The listing builds one solid part. Answer for the finished solid, in the listing's coordinates (mm). A direction names the side the tool comes from. Coordinates: 2 decimals unless noted, no trailing zeros. Order: outer loops, then holes, each group sorted by start corner. A loop starts at its lowest first (then second) coordinate and runs counter-clockwise, first axis right, second up.
```python
from build123d import *

# Parameters (mm, degrees)
SKETCH1_W           = 22.5
SKETCH1_H           = 12.2
BOSS_EXTRUDE1_DEPTH = 3.000000026


with BuildPart() as part:
    # Sketch1 → Boss-Extrude1 (new body)
    with BuildSketch(Plane(origin=(3.000000026, 0, 0), x_dir=(0, 0, -1), z_dir=(1, 0, 0))):
        Polygon((-21.320657805, 14.036174864), (-22.758102044, 12.659284286), (-24.039382115, 11.136000976), (-25.149684399, 9.483940899), (-26.076165959, 7.722207811), (-26.808116585, 5.871174857), (-27.337068692, 3.952247556), (-27.656905353, 1.987616299), (-27.763931081, 0), (-27.656905353, -1.987616299), (-27.337068692, -3.952247556), (-26.808116585, -5.871174857), (-26.076165959, -7.722207811), (-25.149684399, -9.483940899), (-24.039382115, -11.136000976), (-22.758102044, -12.659284286), (-21.320657805, -14.036174864), (-19.743673503, -15.250750817), (-18.045384437, -16.28896594), (-16.245434061, -17.138814554), (-14.364630915, -17.790470272), (-12.424727902, -18.236396834), (-7.814312354, -19.272558391), (-3.327161307, -20.754124969), (0.993806054, -22.666925564), (5.107260309, -24.992663413), (8.973857388, -27.709092945), (12.55661156, -30.790233985), (15.821257606, -34.206613898), (22.763932127, -34.206613898), (22.763932127, -28.999887407), (27.763931084, -28.999887407), (27.763931084, -18.99988763), (22.763932127, -18.99988763), (22.763932127, -12.999887578), (27.763931084, -12.999887578), (27.763931084, -2.999887569), (22.763932127, -2.999887569), (22.763932127, 3.000112483), (27.763931084, 3.000112483), (27.763931084, 13.000112027), (22.763932127, 13.000112027), (22.763932127, 19.00011301), (27.763931084, 19.00011301), (27.763931084, 29.000112787), (22.763932127, 29.000112787), (22.763932127, 34.206613898), (15.821257606, 34.206613898), (12.55661156, 30.790233985), (8.973857388, 27.709092945), (5.107260309, 24.992661551), (0.993806054, 22.666923702), (-3.327161307, 20.754123107), (-7.814312354, 19.272556528), (-12.424727902, 18.236394972), (-14.364630915, 17.790470272), (-16.245434061, 17.138814554), (-18.045384437, 16.28896594), (-19.743673503, 15.250750817), align=None)
        with Locations((-3.903931454, 0.199999778)):
            Rectangle(SKETCH1_W, SKETCH1_H, mode=Mode.SUBTRACT)
        Polygon((-18.119180575, 0.971863221), (-17.898211256, 1.059905044), (-17.663484439, 1.098386711), (-17.425971106, 1.085509197), (-17.196778208, 1.02187437), (-16.986625269, 0.910457922), (-16.891805455, 0.83837827), (-16.728227958, 0.665691623), (-16.605598852, 0.461878022), (-16.529647633, 0.236467487), (-16.503928229, 0), (-16.529647633, -0.236467487), (-16.605598852, -0.461878022), (-16.728227958, -0.665691623), (-16.891805455, -0.83837827), (-16.986625269, -0.910457922), (-17.088681459, -0.971863221), (-17.309648916, -1.059905044), (-17.544377595, -1.098386711), (-17.781890929, -1.085509197), (-18.011083826, -1.02187437), (-18.221236765, -0.910457922), (-18.402526155, -0.756469381), (-18.546473235, -0.567109266), (-18.64635013, -0.351231691), (-18.697483465, -0.118930919), (-18.70393008, 0), (-18.678214401, 0.236467487), (-18.602263182, 0.461878022), (-18.479634076, 0.665691623), (-18.316056579, 0.83837827), align=None, mode=Mode.SUBTRACT)
        Polygon((9.380819276, 0.971863221), (9.601787664, 1.059905044), (9.836516343, 1.098386711), (10.074028745, 1.085509197), (10.303220712, 1.02187437), (10.513374582, 0.910457922), (10.608193465, 0.83837827), (10.771771893, 0.665691623), (10.89440193, 0.461878022), (10.970351286, 0.236467487), (10.996068828, 0), (10.970351286, -0.236467487), (10.89440193, -0.461878022), (10.771771893, -0.665691623), (10.608193465, -0.83837827), (10.513374582, -0.910457922), (10.411318392, -0.971863221), (10.190350004, -1.059905044), (9.955622256, -1.098386711), (9.718108922, -1.085509197), (9.488916956, -1.02187437), (9.278763086, -0.910457922), (9.097473696, -0.756469381), (8.953525685, -0.567109266), (8.853650652, -0.351231691), (8.802517317, -0.118930919), (8.79606884, 0), (8.821786381, 0.236467487), (8.897735737, 0.461878022), (9.020366706, 0.665691623), (9.183944203, 0.83837827), align=None, mode=Mode.SUBTRACT)
    extrude(amount=-BOSS_EXTRUDE1_DEPTH)


solid = part.part
```
(1) Consider line 1 (Y direction, x = 0.8, z = -23); line 2 (Z direction, x = 1.95, y = 0); line 3 (Z direction, x = 1.5, y = 2.5). Determine where each line is inside the solid, lowest interval first.
(2) Find section B-B (z = 4.5). Write down the section's boundary in (x, y).
(3) The mould has two halves that part along Y. Classify faces 4 (the face through (1.521, 21.724, 1.136)), 5 (the face through (2, 3, -25)), 6 (the face through (1.52, -26.33, -7.01)): released by +Y, released by -Y, zero draft, split by the parting line, or undercut.
(4) For faces 1 (the face through (1.521, 13.357, 22.029)), 2 (the face through (2, 0, -22.764)), 3 (the face through (2, 29, -25)), determine the directions among +Z, -Z, +X, -X, +Y, -Y from which every point of the face is accessible in a straight line to the end or side of a thin tool.
(5) Find section D-D (y = -26). Write down the section's boundary in (x, z), and give its area (3 significant figures).
(6) Find section C-C (x = 2.1). Give the number of separate pieces and of enclosed holes in the cut face, and give its area (3 significant figures).
(7) Find section A-A (z = -24). Write down the section's boundary in (x, y), and give its area (3 significant figures).
(8) Each of these flat-tipped pins is pushed along its axis until it touches: pin 1 Ø1.5 at (x, z) = (1.5, 3.5) entering from +Y; pin 2 Ø0.9 at (x, y) = (2, 15.5) entering from -Z; pin 3 Ø1 at (x, z) = (1, 7.5) entering from +Y. Where does it stop, or does it pass through?
Findings below:
1. line 1: y = -29 to -19, -13 to -3, 3 to 13, 19 to 29
1. line 2: z = -22.76 to -11, -8.8 to -7.35, 15.15 to 16.5, 18.7 to 27.76
1. line 3: z = -22.76 to -7.35, 15.15 to 27.57
2. outline: (0, -20.37) - (3, -20.37) - (3, -5.9) - (0, -5.9) - close; (0, 6.3) - (3, 6.3) - (3, 20.37) - (0, 20.37) - close
3. face 4: released by +Y
3. face 5: undercut
3. face 6: released by -Y
4. face 1: +Z, +X, -X, +Y
4. face 2: -Z, +X, -X
4. face 3: -Z, +X, -X, +Y
5. outline: (0, -27.76) - (3, -27.76) - (3, -6.54) - (0, -6.54) - close
5. area: 63.7 mm2
6. separate pieces: 1
6. enclosed holes: 3
6. area: 2,180 mm2
7. outline: (0, -29) - (3, -29) - (3, -19) - (0, -19) - close; (0, -13) - (3, -13) - (3, -3) - (0, -3) - close; (0, 3) - (3, 3) - (3, 13) - (0, 13) - close; (0, 19) - (3, 19) - (3, 29) - (0, 29) - close
7. area: 120 mm2
8. pin 1: stops at y = 21.01
8. pin 2: stops at z = -22.76
8. pin 3: stops at y = 19.54
